```python
from build123d import *

# Parameters (mm, degrees)
SKETCH1_R             = 6
BOSS_EXTRUDE1_DEPTH   = 388
CHAMFER1_SIZE         = 1
M5_TAPPED_HOLE1_D     = 4.2
M5_TAPPED_HOLE1_DEPTH = 14
M5_TAPPED_HOLE1_TIP   = 1.2618073
M5_TAPPED_HOLE2_D     = 4.2
M5_TAPPED_HOLE2_DEPTH = 14
M5_TAPPED_HOLE2_TIP   = 1.2618073


with BuildPart() as part:
    # Sketch1 → Boss-Extrude1 (new body)
    with BuildSketch(Plane(origin=(0, 0, 0), x_dir=(0, 0, -1), z_dir=(1, 0, 0))):
        with Locations(Location((0, 0, 0), (0, 0, 180))):
            Circle(SKETCH1_R)
    extrude(amount=BOSS_EXTRUDE1_DEPTH)

    # Chamfer1
    chamfer1_edges = [part.edges().sort_by_distance(p)[0] for p in [
        (0, 0, -6),
        (388, 0, -6),
    ]]
    chamfer(chamfer1_edges, length=CHAMFER1_SIZE)

    # M5 Tapped Hole1
    with Locations(Plane(origin=(388, 0, 0), x_dir=(0, 0, -1), z_dir=(1, 0, 0))):
        with Locations((0, 0)):
            Hole(M5_TAPPED_HOLE1_D / 2, depth=M5_TAPPED_HOLE1_DEPTH)
            with Locations((0, 0, -(M5_TAPPED_HOLE1_DEPTH + M5_TAPPED_HOLE1_TIP / 2))):  # 118° drill point
                Cone(0, M5_TAPPED_HOLE1_D / 2, M5_TAPPED_HOLE1_TIP, mode=Mode.SUBTRACT)

    # M5 Tapped Hole2
    with Locations(Plane.ZY):
        with Locations((0, 0)):
            Hole(M5_TAPPED_HOLE2_D / 2, depth=M5_TAPPED_HOLE2_DEPTH)
            with Locations((0, 0, -(M5_TAPPED_HOLE2_DEPTH + M5_TAPPED_HOLE2_TIP / 2))):  # 118° drill point
                Cone(0, M5_TAPPED_HOLE2_D / 2, M5_TAPPED_HOLE2_TIP, mode=Mode.SUBTRACT)


solid = part.part
```
Geometry: final body of the model. Coordinates: model frame, mm. Round coordinates to 2 decimals unless told otherwise and drop trailing zeros. Order: outer loops, then holes, each group sorted by start corner. A loop starts at its lowest first (then second) coordinate and runs counter-clockwise, first axis right, second up. Notation, with made-up numbers: M 89.5,24.25 L 106.5,24.25 A15 ccw 106.5,36.25 Z; hole C 20,-16 d10. An arc over 180 degrees is marked long. One line per item, written item: value.
(1) Line query: probe 1 along Y at (x, z) = (9, 0); probe 2 along X at (y, z) = (-2, -0.25); probe 3 along Y at (x, z) = (188.5, -0.75). Output: solid intervals per line, ascending. Write a range as [from, to].
Result sheet:
probe 1: [-6, -2.1], [2.1, 6]
probe 2: [14.05, 373.95]
probe 3: [-5.95, 5.95]
(2) Cut plane A-A (x = 191). Return the cut outline in (y, z).
Result sheet:
outline: C 0,0 d12
(3) Pin query (flat end, axial travel): P1, Ø3, axis at x = 94, z = 3.5, coming from the +Y side; P2, Ø3, axis at y = -1.5, z = -1, coming from the -X side; P3, Ø4, axis at y = 0, z = 0, coming from the +X side; P4, Ø1, axis at x = 320.5, y = -3.5, coming from the -Z side. Return the tip coordinate at first contact, or that it passes through.
Result sheet:
P1: y = 5.66
P2: x = 0
P3: x = 373.94
P4: z = -5.2
